Source: CAD feature listing. Evaluate the final solid. Frame: model axes, mm. Face numbers are marked on the shaded views. A direction names the side the tool comes from. Coordinates: 2 decimals unless noted, no trailing zeros. Write each loop counter-clockwise with the first axis right and the second up, starting at its lowest first coordinate (ties: lowest second). Pieces come first, ordered by that corner, then holes. Notation, with made-up numbers: M 2,71 L 29,71 A23 cw 29,89 Z; hole C -29.75,51.5 d4. An arc over 180 degrees is marked long. Answer as CSV lines item,"result". Start each with the question number.
1. Section B-B on y = 4.75. Return the cut outline in (x, z), plus the area to 3 significant figures.
2. Reachability of the marked faces 1 and 2 from +Z, -Z, +X, -X, +Y, -Y: full face, straight path, thin tool, end or side. Return the list, or none.
3. Mould query, pull axis X, two halves, no side actions, for the marked faces 3, 4, 5 and 6. Classes: pulls with the +X half, pulls with the -X half, needs draft (parallel to the pull), parting line crosses it, or undercut.
4. Section C-C on z = 0. Return the cut outline in (x, y).
5. Section A-A on x = -12.5. Return the cut outline in (y, z), plus the area to 3 significant figures.
6. Line query: probe 1 along Z at (x, y) = (-18, 10.5); probe 2 along X at (y, z) = (15, -7); probe 3 along Y at (x, z) = (17.5, 15.5). Output: solid intervals per line, ascending. Write a range as [from, to].
7. Contact query for a flat-ended pin moving along its axis: pin 1 Ø5 at (x, z) = (7, -9) entering from +Y. Output: stop coordinate, or through.
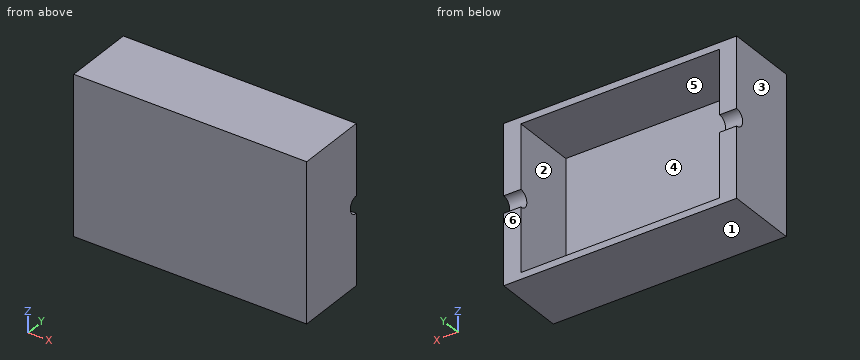
```python
from build123d import *

# Parameters (mm, degrees)
CROQUIS1_W              = 70.8
CROQUIS1_H              = 48
CROQUIS1_W_2            = 60.4
CROQUIS1_H_2            = 44
SALIENTE_EXTRUIR1_DEPTH = 19.6
CROQUIS1_2_W            = 70.8
CROQUIS1_2_H            = 48
CROQUIS1_2_W_2          = 60.4
CROQUIS1_2_H_2          = 44
SALIENTE_EXTRUIR2_DEPTH = 2
CORTAR_EXTRUIR1_REACH   = 79.284


with BuildPart() as part:
    # Croquis1 → Saliente-Extruir1 (new body)
    with BuildSketch(Plane(origin=(0, 0, 0), x_dir=(1, 0, 0), z_dir=(0, 1, 0))):
        Rectangle(CROQUIS1_W, CROQUIS1_H)
        Rectangle(CROQUIS1_W_2, CROQUIS1_H_2, mode=Mode.SUBTRACT)
    extrude(amount=SALIENTE_EXTRUIR1_DEPTH)

    # Croquis1<2> → Saliente-Extruir2 (add)
    # profile 1 of 2: a face of its own
    with BuildSketch(Plane(origin=(0, 0, 0), x_dir=(1, 0, 0), z_dir=(0, 1, 0))):
        Rectangle(CROQUIS1_2_W, CROQUIS1_2_H)
        Rectangle(CROQUIS1_2_W_2, CROQUIS1_2_H_2, mode=Mode.SUBTRACT)
    # profile 2 of 2: a face of its own
    with BuildSketch(Plane(origin=(0, 0, 0), x_dir=(1, 0, 0), z_dir=(0, 1, 0))):
        Rectangle(CROQUIS1_2_W_2, CROQUIS1_2_H_2)
    extrude(amount=-SALIENTE_EXTRUIR2_DEPTH)

    # Cortar-Extruir1: up to this face of the body (flat: up to its plane)
    cortar_extruir1_end = Plane(part.part.faces().sort_by_distance((-35.4, 8.8, 0))[0])
    # Croquis2 → Cortar-Extruir1 (cut, up to the picked face)
    with BuildSketch(Plane(origin=(35.4, 0, 0), x_dir=(0, 0, -1), z_dir=(1, 0, 0)), mode=Mode.PRIVATE) as cortar_extruir1_sk1:
        with BuildLine():
            Line((-2.6, 19.6), (2.6, 19.6))
            ThreePointArc((2.6, 19.6), (0, 17), (-2.6, 19.6))
        make_face()
    cortar_extruir1_tool1 = split(extrude(cortar_extruir1_sk1.sketch, amount=-CORTAR_EXTRUIR1_REACH, mode=Mode.PRIVATE), bisect_by=cortar_extruir1_end, keep=Keep.BOTH, mode=Mode.PRIVATE)
    add(cortar_extruir1_tool1.solids().sort_by(Axis((35.4, 18.496526, 0), (-1, 0, 0)))[0], mode=Mode.SUBTRACT)


solid = part.part
```
Values:
1,outline,"M -35.4,-24 L 35.4,-24 L 35.4,24 L -35.4,24 Z; hole M -30.2,-22 L 30.2,-22 L 30.2,22 L -30.2,22 Z"
1,area,"741 mm²"
2,face 1,"-Z, +X, -X, +Y, -Y"
2,face 2,"+Y"
3,face 3,"pulls with the -X half"
3,face 4,"undercut"
3,face 5,"undercut"
3,face 6,"needs draft"
4,outline,"M -35.4,-2 L 35.4,-2 L 35.4,17 L 30.2,17 L 30.2,0 L -30.2,0 L -30.2,17 L -35.4,17 Z"
5,outline,"M -2,-24 L 19.6,-24 L 19.6,-22 L 0,-22 L 0,22 L 19.6,22 L 19.6,24 L -2,24 Z"
5,area,"174 mm²"
6,probe 1,"[-24, -22], [22, 24]"
6,probe 2,"[-35.4, -30.2], [30.2, 35.4]"
6,probe 3,"[-2, 0]"
7,pin 1,"y = 0"
